Verification items for this drawing (mm, ordinates from the low corner). Round coordinates to 2 decimals unless told otherwise and drop trailing zeros. Write each loop counter-clockwise with the first axis right and the second up, starting at its lowest first coordinate (ties: lowest second). Pieces come first, ordered by that corner, then holes. Notation, with made-up numbers: (-25, 50) -> (18, 50) arc R19 cw to (18, 79) -> close; hole circle Ø7 at (-4, -2.5). An arc over 180 degrees is marked (long way). Put each result on its own line as item: value. Start each with the question number.
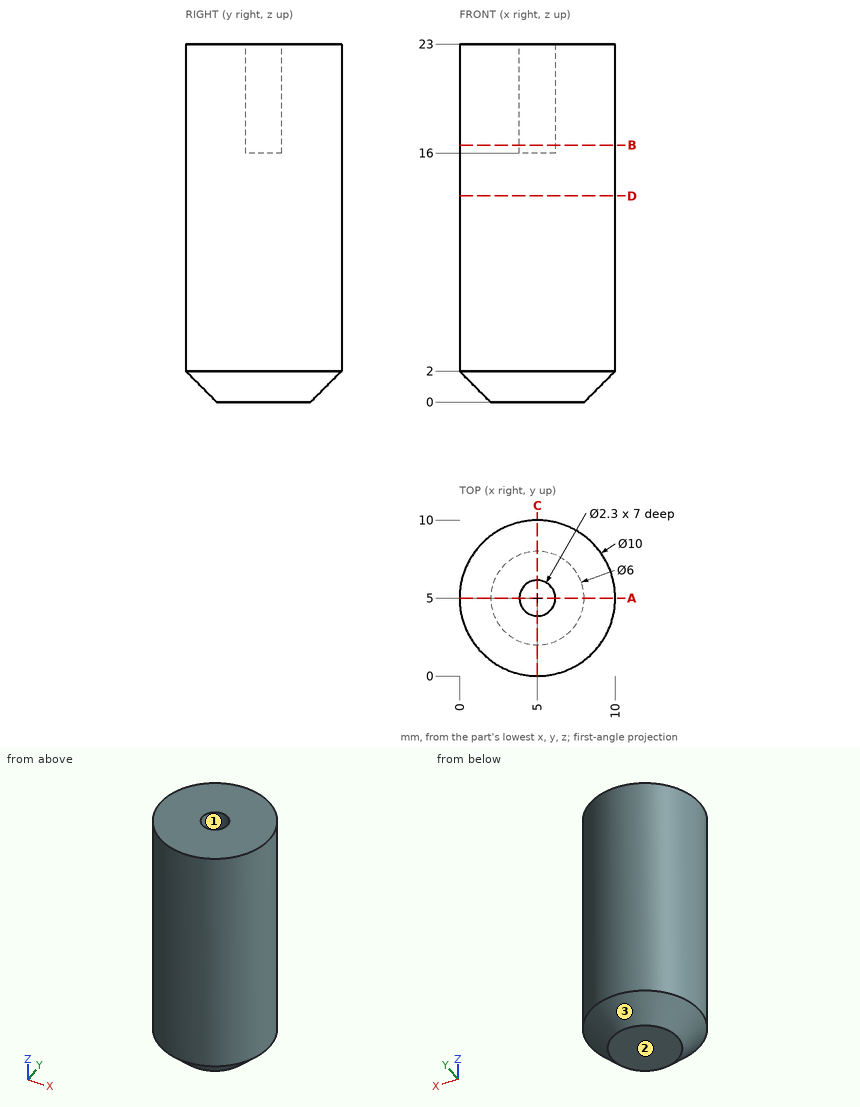
1. Material ranges on L1, parallel to Y at x = 5, z = 20; L2, parallel to Z at x = 5, y = 6; L3, parallel to Y at x = 1, z = 21, recorded low to high. Write a range as [from, to].
2. Gauge pin test, flat ends, axial feed: P1, Ø1, axis at y = 8, z = 14.5, coming from the +X side; P2, Ø1, axis at y = 2.5, z = 3, coming from the -X side. Record the tip position at first contact, or that the pin passes through.
3. Draft check along Y on the marked faces 1, 2 and 3. Enter one of: released by +Y, released by -Y, zero draft, split by the parting line, or undercut.
4. Section check D-D, the plane z = 13.25. Enter the section's corners in (x, y), then the cut area to 3 significant figures.
5. Section check A-A, the plane y = 5. Enter the section's corners in (x, z), then the cut area to 3 significant figures.
6. Section check B-B, the plane z = 16.5. Enter the section's corners in (x, y).
Reply:
1. L1: y = [0, 3.85], [6.15, 10]
1. L2: z = [0, 16]
1. L3: y = [2, 8]
2. P1: stops at x = 9.33
2. P2: stops at x = 0.42
3. face 1: undercut
3. face 2: zero draft
3. face 3: split by the parting line
4. outline: circle Ø10 at (5, 5)
4. area: 78.5 mm2
5. outline: (0, 2) -> (2, 0) -> (8, 0) -> (10, 2) -> (10, 23) -> (6.15, 23) -> (6.15, 16) -> (3.85, 16) -> (3.85, 23) -> (0, 23) -> close
5. area: 210 mm2
6. outline: circle Ø10 at (5, 5); hole circle Ø2.3 at (5, 5)
